```python
from build123d import *

# Parameters (mm, degrees)
SKETCH_1_W          = 60
SKETCH_1_H          = 50
EXTRUDE_1_DEPTH     = 3
SKETCH_2_R          = 1.25
CUT_EXTRUDE_1_DEPTH = 3
SKETCH_4_W          = 3
SKETCH_4_H          = 28
EXTRUDE_3_DEPTH     = 60
SKETCH_5_W          = 44
SKETCH_5_H          = 28
CUT_EXTRUDE_2_DEPTH = 10
EXTRUDE_4_DEPTH     = 3
SKETCH_8_R          = 2.1
CUT_EXTRUDE_3_DEPTH = 65.288412642
EXTRUDE_5_DEPTH     = 60
SKETCH_9_W          = 10
SKETCH_9_H          = 20
SKETCH_9_W_2        = 28
CUT_EXTRUDE_4_DEPTH = 54.293490307
SKETCH_11_R         = 1.6
CUT_EXTRUDE_5_DEPTH = 54.293490307
SKETCH_12_W         = 1.537741429
SKETCH_12_H         = 3
CUT_EXTRUDE_6_DEPTH = 72.413687212
FILLET_1_R          = 8
FILLET_2_R          = 8
FILLET_3_R          = 3
FILLET_4_R          = 3
FILLET_5_R          = 2
RIB_2_REACH         = 77.736
SKETCH_14_WALL_W    = 171.36018765
SKETCH_14_WALL_H    = 3
RIB_3_REACH         = 77.736
SKETCH_16_WALL_W    = 171.36018765
SKETCH_16_WALL_H    = 3
RIB_4_REACH         = 71.346
SKETCH_17_WALL_W    = 148.898052794
SKETCH_17_WALL_H    = 2
RIB_5_REACH         = 71.346
SKETCH_18_WALL_W    = 148.810340372
SKETCH_18_WALL_H    = 2


with BuildPart() as part:
    # 草图1 → 凸台-拉伸1 (new body)
    with BuildSketch(Plane(origin=(0, 0, 0), x_dir=(1, 0, 0), z_dir=(0, 1, 0))):
        Rectangle(SKETCH_1_W, SKETCH_1_H)
    extrude(amount=EXTRUDE_1_DEPTH)

    # 草图2 → 切除-拉伸1 (cut)
    with BuildSketch(Plane(origin=(0, 3, 0), x_dir=(1, 0, 0), z_dir=(0, 1, 0))):
        with Locations(Location((-14.000714267, -14.000714267, 0), (0, 0, 270))):
            Circle(SKETCH_2_R)
        with Locations(Location((14.000714267, 14.000714267, 0), (0, 0, 270))):
            Circle(SKETCH_2_R)
    extrude(amount=-CUT_EXTRUDE_1_DEPTH, mode=Mode.SUBTRACT)

    # 草图4 → 凸台-拉伸3 (add)
    with BuildSketch(Plane(origin=(30, 0, 0), x_dir=(0, 0, -1), z_dir=(1, 0, 0))):
        with Locations((23.5, -14)):
            Rectangle(SKETCH_4_W, SKETCH_4_H)
    extrude(amount=-EXTRUDE_3_DEPTH)

    # 草图5 → 切除-拉伸2 (cut)
    with BuildSketch(Plane(origin=(0, 0, -25), x_dir=(-1, 0, 0), z_dir=(0, 0, -1))):
        with Locations((0, -14)):
            Rectangle(SKETCH_5_W, SKETCH_5_H)
    extrude(amount=-CUT_EXTRUDE_2_DEPTH, mode=Mode.SUBTRACT)

    # 草图7 → 凸台-拉伸4 (add)
    with BuildSketch(Plane.XY.offset(-22)):
        with BuildLine():
            Line((-30, -28), (-22, -28))
            ThreePointArc((-22, -28), (-26, -32), (-30, -28))
        make_face()
        with BuildLine():
            Line((22, -28), (30, -28))
            ThreePointArc((30, -28), (26, -32), (22, -28))
        make_face()
    extrude(amount=-EXTRUDE_4_DEPTH)

    # 草图8 → 切除-拉伸3 (cut, through all)
    with BuildSketch(Plane.XY.offset(-22)):
        with Locations((26, -28)):
            Circle(SKETCH_8_R)
        with Locations((-26, -28)):
            Circle(SKETCH_8_R)
    extrude(amount=-CUT_EXTRUDE_3_DEPTH, mode=Mode.SUBTRACT)

    # 草图3 → 凸台-拉伸5 (add)
    with BuildSketch(Plane(origin=(30, 0, 0), x_dir=(0, 0, -1), z_dir=(1, 0, 0))):
        Polygon((-20.756443745, 0), (-32.524054991, -12.913843028), (-39.697792397, -12.913843028), (-39.697792397, -10.913843028), (-33.407389674, -10.913843028), (-23.462258571, 0), align=None)
    extrude(amount=-EXTRUDE_5_DEPTH)

    # 草图9 → 切除-拉伸4 (cut, through all)
    with BuildSketch(Plane.XZ.offset(12.913843028)):
        with Locations((25, 29.697792397)):
            Rectangle(SKETCH_9_W, SKETCH_9_H)
        with Locations((0, 29.697792397)):
            Rectangle(SKETCH_9_W_2, SKETCH_9_H)
        with Locations((-25, 29.697792397)):
            Rectangle(SKETCH_9_W, SKETCH_9_H)
    extrude(amount=-CUT_EXTRUDE_4_DEPTH, mode=Mode.SUBTRACT)

    # 草图11 → 切除-拉伸5 (cut, through all)
    with BuildSketch(Plane.XZ.offset(12.913843028)):
        with Locations(Location((17, 37, 0), (0, 0, 270))):
            Circle(SKETCH_11_R)
        with Locations(Location((-17, 37, 0), (0, 0, 270))):
            Circle(SKETCH_11_R)
    extrude(amount=-CUT_EXTRUDE_5_DEPTH, mode=Mode.SUBTRACT)

    # 草图12 → 切除-拉伸6 (cut, through all)
    with BuildSketch(Plane(origin=(20, 0, 0), x_dir=(0, 0, -1), z_dir=(1, 0, 0))):
        with Locations((-24.231129286, 1.5)):
            Rectangle(SKETCH_12_W, SKETCH_12_H)
    extrude(amount=-CUT_EXTRUDE_6_DEPTH, mode=Mode.SUBTRACT)

    # 圆角1
    fillet_1_edges = [part.edges().sort_by_distance(p)[0] for p in [
        (30, 1.5, 19.697792397),
    ]]
    fillet(fillet_1_edges, radius=FILLET_1_R)

    # 圆角2
    fillet_2_edges = [part.edges().sort_by_distance(p)[0] for p in [
        (-30, 1.5, 19.697792397),
    ]]
    fillet(fillet_2_edges, radius=FILLET_2_R)

    # 圆角3
    fillet_3_edges = [part.edges().sort_by_distance(p)[0] for p in [
        (17, 3, 23.462258571),
        (-17, 3, 23.462258571),
    ]]
    fillet(fillet_3_edges, radius=FILLET_3_R - 0.0001)  # a hair under: the kernel refuses the full size

    # 圆角4
    fillet_4_edges = [part.edges().sort_by_distance(p)[0] for p in [
        (-17, -10.913843028, 33.407389674),
        (17, -10.913843028, 33.407389674),
        (-17, -12.913843028, 32.524054991),
        (17, -12.913843028, 32.524054991),
    ]]
    fillet(fillet_4_edges, radius=FILLET_4_R)

    # 圆角5
    fillet_5_edges = [part.edges().sort_by_distance(p)[0] for p in [
        (0, 3, -25),
    ]]
    fillet(fillet_5_edges, radius=FILLET_5_R)

    # 草图14 wall → 筋2 (add, up to next)
    with BuildSketch(Plane(origin=(26, -8, -18), x_dir=(0, -0.894427191, -0.4472135955), z_dir=(0, 0.4472135955, -0.894427191)), mode=Mode.PRIVATE) as rib_2_sk1:
        Rectangle(SKETCH_14_WALL_W, SKETCH_14_WALL_H)
    rib_2_tool1 = extrude(rib_2_sk1.sketch, amount=RIB_2_REACH, mode=Mode.PRIVATE) - part.part
    add(rib_2_tool1.solids().sort_by_distance((26, -8, -18))[0])

    # 草图16 wall → 筋3 (add, up to next)
    with BuildSketch(Plane(origin=(-26, -8, -18), x_dir=(0, -0.894427191, -0.4472135955), z_dir=(0, -0.4472135955, 0.894427191)), mode=Mode.PRIVATE) as rib_3_sk1:
        Rectangle(SKETCH_16_WALL_W, SKETCH_16_WALL_H)
    rib_3_tool1 = extrude(rib_3_sk1.sketch, amount=-RIB_3_REACH, mode=Mode.PRIVATE) - part.part
    add(rib_3_tool1.solids().sort_by_distance((-26, -8, -18))[0])

    # 草图17 wall → 筋4 (add, up to next)
    with BuildSketch(Plane(origin=(17, -2.393367573, 21.786066703), x_dir=(0, 0.583365802334, -0.81220954234), z_dir=(0, 0.81220954234, 0.583365802334)), mode=Mode.PRIVATE) as rib_4_sk1:
        Rectangle(SKETCH_17_WALL_W, SKETCH_17_WALL_H)
    rib_4_tool1 = extrude(rib_4_sk1.sketch, amount=RIB_4_REACH, mode=Mode.PRIVATE) - part.part
    add(rib_4_tool1.solids().sort_by_distance((17, -2.393367573, 21.786066703))[0])

    # 草图18 wall → 筋5 (add, up to next)
    with BuildSketch(Plane(origin=(-17, -2.360222573, 21.75586365), x_dir=(0, -0.581503003153, 0.813544256525), z_dir=(0, 0.813544256525, 0.581503003153)), mode=Mode.PRIVATE) as rib_5_sk1:
        Rectangle(SKETCH_18_WALL_W, SKETCH_18_WALL_H)
    rib_5_tool1 = extrude(rib_5_sk1.sketch, amount=RIB_5_REACH, mode=Mode.PRIVATE) - part.part
    add(rib_5_tool1.solids().sort_by_distance((-17, -2.360222573, 21.75586365))[0])


solid = part.part
```
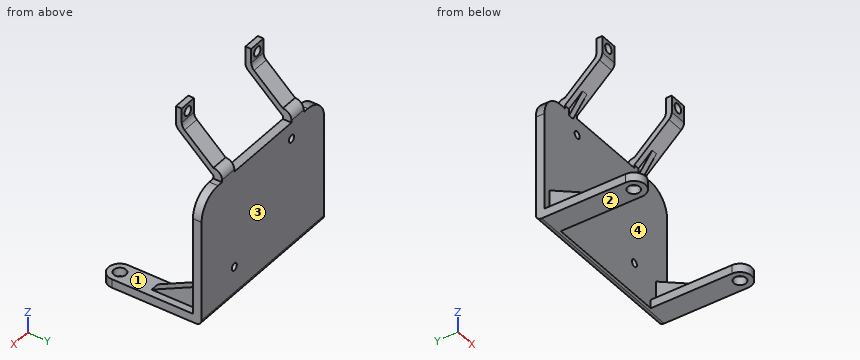
The listing builds one solid part. Answer for the finished solid, in the listing's coordinates (mm). Face numbers are marked on the shaded views. A direction names the side the tool comes from. Coordinates: 2 decimals unless noted, no trailing zeros. Loops run counter-clockwise (first coordinate to the right, second up) from the corner with the lowest first, then second, coordinate; pieces in that order, holes last. Notation, with made-up numbers: M 26,23.25 L 76,23.25 A21 cw 76,60.25 Z; hole C 2,42.25 d6. An arc over 180 degrees is marked long. Answer as CSV lines item,"result". Start each with the question number.
(1) The part is cut by section A-A (z = 37). Give the vertices of the cut face in (x, y).
(2) Find the intervals of material crossed by L1, parallel to X at y = -11, z = 37; L2, parallel to X at y = -5.5, z = -21; L3, parallel to Y at x = 18, z = 7, in increasing order. Write a range as [from, to].
(3) The mould has two halves that part along X. Classify the marked faces 3 and 4: pulls with the +X half, pulls with the -X half, needs draft (parallel to the pull), parting line crosses it, or undercut.
(4) For the marked faces 1 and 2, determine the directions among +Z, -Z, +X, -X, +Y, -Y from which every point of the face is accessible in a straight line to the end or side of a thin tool.
(5) The part is cut by section B-B (y = -17.5). Give the vertices of the cut face in (x, z), and give its area (3 significant figures).
(6) The part is cut by section D-D (z = -16.5). Give the vertices of the cut face in (x, y).
(7) Given pin 1 (5.5 mm diameter, centred on x = 18.5, z = 36.5, fed in from +Y); pin 2 (12 mm diameter, centred on x = 22.5, z = 26.5, fed in from -Y); pin 3 (1.8 mm diameter, centred on x = 16.5, z = 38, fed in from -Y), each flat-ended and moving along its own axis, determine where each tip first touches the part or whether it passes through.
Determined:
1,outline,"M -20,-12.91 L -18.6,-12.91 L -18.6,-10.91 L -20,-10.91 Z; M -15.4,-12.91 L -14,-12.91 L -14,-10.91 L -15.4,-10.91 Z; M 14,-12.91 L 15.4,-12.91 L 15.4,-10.91 L 14,-10.91 Z; M 18.6,-12.91 L 20,-12.91 L 20,-10.91 L 18.6,-10.91 Z"
2,L1,"[-20, -18.6], [-15.4, -14], [14, 15.4], [18.6, 20]"
2,L2,"[-27.5, -24.5], [24.5, 27.5]"
2,L3,"[0, 3]"
3,face 3,"needs draft"
3,face 4,"undercut"
4,face 1,"+Z, -Y"
4,face 2,"-Z, +X, -X, +Y, -Y"
5,outline,"M -30,-25 L -22,-25 L -22,-22 L -30,-22 Z; M 22,-25 L 30,-25 L 30,-22 L 22,-22 Z"
5,area,"48.0 mm2"
6,outline,"M -30,0 L -27.5,0 L -27.5,-5 L -24.5,-5 L -24.5,0 L 24.5,0 L 24.5,-5 L 27.5,-5 L 27.5,0 L 30,0 L 30,3 L -30,3 Z"
7,pin 1,"y = -10.75"
7,pin 2,"y = -12.24"
7,pin 3,"y = -12.91"
